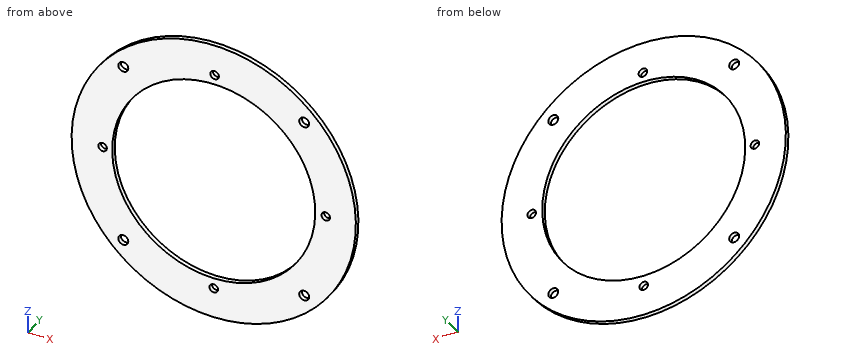
```python
from build123d import *

# Parameters (mm, degrees)
SKETCH1_R           = 50
SKETCH1_R_2         = 35.715
BOSS_EXTRUDE1_DEPTH = 1.59
SKETCH2_R           = 1.5
CUT_EXTRUDE1_DEPTH  = 2
SKETCH3_R           = 1.75
CUT_EXTRUDE2_DEPTH  = 2


with BuildPart() as part:
    # Sketch1 → Boss-Extrude1 (new body)
    with BuildSketch(Plane(origin=(0, 0, 0), x_dir=(1, 0, 0), z_dir=(0, 1, 0))):
        with Locations(Location((0, 0, 0), (0, 0, 90))):
            Circle(SKETCH1_R)
        with Locations(Location((0, 0, 0), (0, 0, 90))):
            Circle(SKETCH1_R_2, mode=Mode.SUBTRACT)
    extrude(amount=BOSS_EXTRUDE1_DEPTH)

    # Sketch2 → Cut-Extrude1 (cut)
    with BuildSketch(Plane(origin=(0, 1.59, 0), x_dir=(1, 0, 0), z_dir=(0, 1, 0))):
        with Locations(Location((0, 39.4, 0), (0, 0, 270))):
            Circle(SKETCH2_R)
        with Locations(Location((39.4, 0.3, 0), (0, 0, 270))):
            Circle(SKETCH2_R)
        with Locations(Location((0.3, -39.1, 0), (0, 0, 270))):
            Circle(SKETCH2_R)
        with Locations(Location((-39.1, 0, 0), (0, 0, 270))):
            Circle(SKETCH2_R)
    extrude(amount=-CUT_EXTRUDE1_DEPTH, mode=Mode.SUBTRACT)

    # Sketch3 → Cut-Extrude2 (cut)
    with BuildSketch(Plane(origin=(0, 1.59, 0), x_dir=(1, 0, 0), z_dir=(0, 1, 0))):
        with Locations(Location((-31.8198, 31.819810307, 0), (0, 0, 270))):
            Circle(SKETCH3_R)
        with Locations(Location((31.819810307, 31.8198, 0), (0, 0, 270))):
            Circle(SKETCH3_R)
        with Locations(Location((31.8198, -31.819810307, 0), (0, 0, 270))):
            Circle(SKETCH3_R)
        with Locations(Location((-31.819810307, -31.8198, 0), (0, 0, 270))):
            Circle(SKETCH3_R)
    extrude(amount=-CUT_EXTRUDE2_DEPTH, mode=Mode.SUBTRACT)


solid = part.part
```
Input: part model. Units: mm. Frame: model coordinates. Round coordinates to 2 decimals unless told otherwise and drop trailing zeros. Loops run counter-clockwise (first coordinate to the right, second up) from the corner with the lowest first, then second, coordinate; pieces in that order, holes last.
1) Pin query (flat end, axial travel): pin 1 (4 mm diameter, centred on x = 31.82, z = 31.82, fed in from +Y). Return the tip coordinate at first contact, or that it passes through.
Ans:
pin 1: stops at y = 1.59
2) Section query A-A on z = -18. Return the cut outline in (x, y).
Ans:
outline: (-46.65, 0) - (-30.85, 0) - (-30.85, 1.59) - (-46.65, 1.59) - close; (30.85, 0) - (46.65, 0) - (46.65, 1.59) - (30.85, 1.59) - close
3) Section query C-C on z = -0.3. Return the cut outline in (x, y), plus the area to 3 significant figures.
Ans:
outline: (-50, 0) - (-40.57, 0) - (-40.57, 1.59) - (-50, 1.59) - close; (-37.63, 0) - (-35.71, 0) - (-35.71, 1.59) - (-37.63, 1.59) - close; (35.71, 0) - (37.9, 0) - (37.9, 1.59) - (35.71, 1.59) - close; (40.9, 0) - (50, 0) - (50, 1.59) - (40.9, 1.59) - close
area: 36.0 mm2
4) Section query B-B on x = 12. Return the cut outline in (y, z), plus the area to 3 significant figures.
Ans:
outline: (0, -48.54) - (1.59, -48.54) - (1.59, -33.64) - (0, -33.64) - close; (0, 33.64) - (1.59, 33.64) - (1.59, 48.54) - (0, 48.54) - close
area: 47.4 mm2
5) Material intervals for line 1 (X direction, y = 1.15, z = -31); line 2 (Z direction, x = -31.5, y = 1.2); line 3 (X direction, y = 0.4, z = 0.5), sorted ascending.
Ans:
line 1: x = -39.23 to -33.37, -30.27 to -17.74, 17.74 to 30.27, 33.37 to 39.23
line 2: z = -38.83 to -33.54, -30.1 to -16.83, 16.83 to 30.1, 33.54 to 38.83
line 3: x = -50 to -40.51, -37.69 to -35.71, 35.71 to 38.13, 40.67 to 50
6) Section query D-D on y = 0.9. Count the separate pieces of the cut face and the enclosed holes in it, plus the area to 3 significant figures.
Ans:
separate pieces: 1
enclosed holes: 9
area: 3,780 mm2
